```python
from build123d import *

# Parameters (mm, degrees)
F0_W      = 8.9
F0_H      = 50
F1_DEPTH  = 7.5
F2_W      = 43
F2_H      = 43
F3_DEPTH  = 6
F4_W      = 8.9
F4_H      = 9
F5_DEPTH  = 4.5
F6_R      = 4.49999
F7_R      = 1.95
F8_DEPTH  = 1.8
F9_R      = 1.95
F10_DEPTH = 1.8
F12_D     = 3.3
F13_R     = 1.75


# Not quite as in the source:
# - a fillet or chamfer is up to 0.001 mm smaller than in the source, because OpenCascade refuses the exact size
# - a feature names something its author has since deleted; it is built from what else it names


with BuildPart() as f1:
    # F0 (on Top) → F1 (new body)
    with BuildSketch(Plane.XY):
        Polygon((-4.45, -9.0662492651), (-24, -9.0662492651), (-24, -57.0662492651), (24, -57.0662492651), (24, -9.0662492651), (4.45, -9.0662492651), align=None)
        with Locations((0, 15.9337507349)):
            Rectangle(F0_W, F0_H)
    extrude(amount=F1_DEPTH)

    # F2 (on face) → F3 (cut)
    with BuildSketch(Plane.XY.offset(7.5)):
        with Locations((0, -33.0662492651)):
            Rectangle(F2_W, F2_H)
    extrude(amount=-F3_DEPTH, mode=Mode.SUBTRACT)

    # F4 (on face) → F5 (join)
    with BuildSketch(Plane.XY.offset(7.5)):
        with Locations((0, 36.4337507349)):
            Rectangle(F4_W, F4_H)
    extrude(amount=F5_DEPTH)

    # F6 (radius 4.5 in the source; OpenCascade refuses exactly that, so slightly less here)
    f6_edges = [f1.edges().sort_by_distance(p)[0] for p in [
        (0, 40.933751, 12),
        (0, 31.933751, 12),
    ]]
    fillet(f6_edges, radius=F6_R)

    # F7 (on face) → F8 (join)
    with BuildSketch(Plane(origin=(21.5, 0, 0), x_dir=(0, -1, 0), z_dir=(-1, 0, 0))):
        with Locations((33.0662492651, 4.5)):
            Circle(F7_R)
    extrude(amount=F8_DEPTH)

    # F9 (on face) → F10 (join)
    with BuildSketch(Plane.YZ.offset(-21.5)):
        with Locations((-33.0662492651, 4.5)):
            Circle(F9_R)
    extrude(amount=F10_DEPTH)

    # F12 (through all)
    with Locations(Plane.YZ.offset(4.45)):
        with Locations((36.4337507349, 7)):
            Hole(F12_D / 2)

    # F13
    f13_edges = [f1.edges().sort_by_distance(p)[0] for p in [
        (-19.7, -35.016249, 4.5),
        (19.7, -31.116249, 4.5),
    ]]
    fillet(f13_edges, radius=F13_R)


solid = f1.part
```
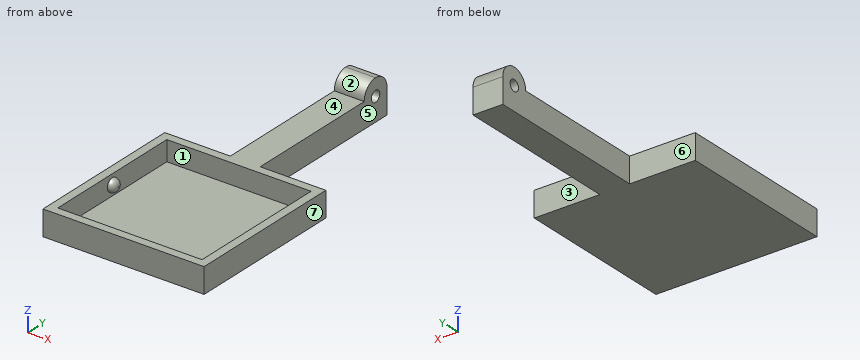
Geometry: final body of the model. Coordinates: model frame, mm. Face numbers are marked on the shaded views. A direction names the side the tool comes from. Give positions to 0.01 mm unless a question says otherwise; leave off trailing zeros. Write each loop counter-clockwise with the first axis right and the second up, starting at its lowest first coordinate (ties: lowest second). Pieces come first, ordered by that corner, then holes.
1. Section query C-C, the plane y = -2.5. Return loops of the section in (x, z), then the cut area to 4 significant figures.
2. Pin query (flat end, axial travel): P1, Ø14.5, axis at x = 6, y = -31, coming from the +Z side; P2, Ø4.5, axis at y = 36.43, z = 7, coming from the -X side; P3, Ø4, axis at x = -12, z = 8.5, coming from the +Y side. Return the tip coordinate at first contact, or that it passes through.
3. Section query D-D, the plane z = 11. Return loops of the section in (x, y).
4. Draft query along Y for the marked faces 1, 2, 3 and 4. Return one class per face: released by +Y, released by -Y, zero draft, split by the parting line, or undercut.
5. Section query B-B, the plane x = -13.5. Return loops of the section in (y, z).
6. Reachability of the marked faces 5, 6 and 7 from +Z, -Z, +X, -X, +Y, -Y: full face, straight path, thin tool, end or side. Return the list, or none.
7. Line query: probe 1 along Y at (x, z) = (-8, 5.5); probe 2 along X at (y, z) = (-35.5, 4.75); probe 3 along Y at (x, z) = (1, 3). Output: solid intervals per line, ascending.
Computed:
1. outline: (-4.45, 0) - (4.45, 0) - (4.45, 7.5) - (-4.45, 7.5) - close
1. area: 66.75 mm2
2. P1: stops at z = 1.5
2. P2: stops at x = -4.45
2. P3: stops at y = -9.07
3. outline: (-4.45, 33.61) - (4.45, 33.61) - (4.45, 39.26) - (-4.45, 39.26) - close
4. face 1: undercut
4. face 2: released by -Y
4. face 3: released by +Y
4. face 4: zero draft
5. outline: (-57.07, 0) - (-9.07, 0) - (-9.07, 7.5) - (-11.57, 7.5) - (-11.57, 1.5) - (-54.57, 1.5) - (-54.57, 7.5) - (-57.07, 7.5) - close
6. face 5: +Z, -Z, +X, +Y
6. face 6: +Z, -Z, -X, +Y
6. face 7: +Z, -Z, +X, +Y, -Y
7. probe 1: y = -57.07 to -54.57, -11.57 to -9.07
7. probe 2: x = -24 to -21.5, 21.5 to 24
7. probe 3: y = -57.07 to -54.57, -11.57 to 40.93
